Read the model definition and answer for the solid it produces. Units are mm, in the model's axes. Give positions to 0.01 mm unless a question says otherwise; leave off trailing zeros. Order: outer loops, then holes, each group sorted by start corner. A loop starts at its lowest first (then second) coordinate and runs counter-clockwise, first axis right, second up. Notation, with made-up numbers: (20.25, -7) -> (24.25, -7) arc R15 ccw to (24.25, 7) -> close; hole circle Ø8 at (-32.5, 0). An arc over 180 degrees is marked (long way). Use one line per item in the form item = value.
```python
from build123d import *

# Parameters (mm, degrees)
F0_R     = 5.1
F0_R_2   = 3
F1_DEPTH = 10
F2_R     = 5
F2_R_2   = 3
F3_DEPTH = 15
F3_TAPER = 3


with BuildPart() as f1:
    # F0 (on Top) → F1 (new body)
    with BuildSketch(Plane.XY):
        Circle(F0_R)
        Circle(F0_R_2, mode=Mode.SUBTRACT)
    extrude(amount=F1_DEPTH)

    # F2 (on face) → F3 (join)
    with BuildSketch(Plane.XY.offset(10)):
        Circle(F2_R)
        Circle(F2_R_2, mode=Mode.SUBTRACT)
    extrude(amount=F3_DEPTH, taper=F3_TAPER)


solid = f1.part
```
Item 1: Straight lines are drawn through the part: L1, parallel to Y at x = 0, z = 4.25; L2, parallel to X at y = 3, z = 17.5; L3, parallel to X at y = -0.5, z = 2.5. For each, find the intervals that lie inside material, in ascending order. Write a range as from..to.
Checks:
L1 = -5.1..-3, 3..5.1
L2 = -3.5..-1.59, 1.59..3.5
L3 = -5.08..-2.96, 2.96..5.08
Item 2: The part is cut by section C-C on z = 11.75. Give the vertices of the cut face in (x, y).
Checks:
outline = circle Ø9.82 at (0, 0); hole circle Ø6.18 at (0, 0)
Item 3: Determine the mould class of faces 1 (the conical face through (-0.737, 3.318, 17.605)), 2 (the cylindrical face through (2.4, -4.5, 4.9)), 3 (the flat face through (3.3, 0.1, 0)) for opening direction Y: +Y half, -Y half, draft (parallel to the pull), parting line (faces both ways), or undercut.
Checks:
face_1 = undercut
face_2 = parting line
face_3 = draft
Item 4: The part is cut by section B-B on z = 7.25. Give the vertices of the cut face in (x, y).
Checks:
outline = circle Ø10.2 at (0, 0); hole circle Ø6 at (0, 0)
Item 5: The part is cut by section A-A on x = 0. Give the vertices of the cut face in (y, z).
Checks:
outline = (-5.1, 0) -> (-3, 0) -> (-3, 10) -> (-3.79, 25) -> (-4.21, 25) -> (-5, 10) -> (-5.1, 10) -> close; (3, 0) -> (5.1, 0) -> (5.1, 10) -> (5, 10) -> (4.21, 25) -> (3.79, 25) -> (3, 10) -> close
Item 6: Given pin 1 Ø3 at (y, z) = (-0.5, 12.5) entering from -X; pin 2 Ø3 at (x, z) = (4, 4.5) entering from -Y; pin 3 Ø2 at (y, z) = (0, 22.5) entering from -X; pin 4 Ø3.5 at (x, y) = (0, 0) entering from -Z, each flat-ended and moving along its own axis, determine where each tip first touches the part or whether it passes through.
Checks:
pin_1 = -4.94
pin_2 = -4.45
pin_3 = -4.4
pin_4 = through
